from build123d import *
from OCP.BRepFilletAPI import BRepFilletAPI_MakeChamfer

# Parameters (mm, degrees)
SKETCH1_R           = 1.5
BOSS_EXTRUDE1_DEPTH = 3
BOSS_EXTRUDE2_START = 22.5
SKETCH2_W           = 3.5
SKETCH2_H           = 6
BOSS_EXTRUDE2_DEPTH = 29
SKETCH4_R           = 1.5
BOSS_EXTRUDE5_DEPTH = 1
CHAMFER2_SIZE       = 2
CHAMFER2_SIZE2      = 3.464101615
SKETCH3_W           = 24
SKETCH3_H           = 29
SKETCH3_R           = 11
BOSS_EXTRUDE4_DEPTH = 7
CHAMFER3_SIZE       = 2
MIRROR1_START       = 18
MIRROR1_OUTLINE_R   = 1.5
MIRROR1_DEPTH       = 4
MIRROR1_START_2     = -12
MIRROR1_2_DEPTH     = 6
MIRROR1_START_3     = 6
MIRROR1_3_DEPTH     = 6
MIRROR1_START_4     = 25.102290732
MIRROR1_4_OUTLINE_W = 2
MIRROR1_4_OUTLINE_H = 18.102290732
MIRROR1_4_DEPTH     = 1.897709268
MIRROR1_START_5     = 7.071067812
MIRROR1_5_OUTLINE_W = 2
MIRROR1_5_OUTLINE_H = 2.897709268
MIRROR1_5_DEPTH     = 3.889087296


with BuildPart() as part:
    # Sketch1 → Boss-Extrude1 (new body)
    with BuildSketch(Plane(origin=(0, 0, 0), x_dir=(1, 0, 0), z_dir=(0, 1, 0))):
        Polygon((-6, 17), (-3, 20), (3, 20), (6, 17), (6, -17), (3, -20), (-3, -20), (-6, -17), align=None)
        with Locations(Location((0, 14, 0), (0, 0, 270))):
            Circle(SKETCH1_R, mode=Mode.SUBTRACT)
        with Locations(Location((0, -14, 0), (0, 0, 270))):
            Circle(SKETCH1_R, mode=Mode.SUBTRACT)
    extrude(amount=BOSS_EXTRUDE1_DEPTH)

    # Sketch2 → Boss-Extrude2 (add)
    with BuildSketch(Plane(origin=(0, 3, 0), x_dir=(1, 0, 0), z_dir=(0, 1, 0)).offset(BOSS_EXTRUDE2_START)):
        with Locations((-7.75, 9)):
            Rectangle(SKETCH2_W, SKETCH2_H)
        with Locations((-7.75, -9)):
            Rectangle(SKETCH2_W, SKETCH2_H)
    extrude(amount=-BOSS_EXTRUDE2_DEPTH)

    # Sketch4 → Boss-Extrude5 (add)
    with BuildSketch(Plane(origin=(0, 3, 0), x_dir=(1, 0, 0), z_dir=(0, 1, 0))):
        Polygon((-3, 20), (-6, 17), (-6, 12), (-6, 6), (-6, -6), (-6, -12), (-6, -17), (-3, -20), (3, -20), (6, -17), (6, 17), (3, 20), align=None)
        with Locations(Location((0, 14, 0), (0, 0, 270))):
            Circle(SKETCH4_R, mode=Mode.SUBTRACT)
        with Locations(Location((0, -14, 0), (0, 0, 270))):
            Circle(SKETCH4_R, mode=Mode.SUBTRACT)
    extrude(amount=BOSS_EXTRUDE5_DEPTH)

    # Chamfer2: one chamfer whose edges measure the first distance from different faces: ONE call of the kernel's chamfer builder (chamfer() names one face for all edges)
    chamfer2_edges_1 = [part.edges().sort_by_distance(p)[0] for p in [
        (-6, 0, -9),
        (-6, 0, 9),
    ]]
    chamfer2_side_1 = [part.faces().sort_by_distance(p)[0] for p in [
        (0, 0, 0),
    ]]
    chamfer2_edges_2 = [part.edges().sort_by_distance(p)[0] for p in [
        (-6, 4, -9),
        (-6, 4, 9),
    ]]
    chamfer2_side_2 = [part.faces().sort_by_distance(p)[0] for p in [
        (0, 4, 0),
    ]]
    chamfer2 = BRepFilletAPI_MakeChamfer(part.part.solid().wrapped)
    for e in chamfer2_edges_1:
        chamfer2.Add(CHAMFER2_SIZE, CHAMFER2_SIZE2, e.wrapped, chamfer2_side_1[0].wrapped)  # the first distance lies on this face
    for e in chamfer2_edges_2:
        chamfer2.Add(CHAMFER2_SIZE, CHAMFER2_SIZE2, e.wrapped, chamfer2_side_2[0].wrapped)  # the first distance lies on this face
    add(Compound.cast(chamfer2.Shape()), mode=Mode.REPLACE)

    # Sketch3 → Boss-Extrude4 (add)
    with BuildSketch(Plane.ZY.offset(9.5)):
        with Locations((0, 11)):
            Rectangle(SKETCH3_W, SKETCH3_H)
        with Locations(Location((0, 11, 0), (0, 0, 236.944268849))):
            Circle(SKETCH3_R, mode=Mode.SUBTRACT)
    extrude(amount=BOSS_EXTRUDE4_DEPTH)

    # Chamfer3
    chamfer3_edges = [part.edges().sort_by_distance(p)[0] for p in [
        (-11.25, 25.5, -12),
        (-11.25, -3.5, -12),
        (-11.25, -3.5, 12),
        (-11.25, 25.5, 12),
    ]]
    chamfer(chamfer3_edges, length=CHAMFER3_SIZE)

    # Mirror1: read off the stored shape, not the designer's step
    # Mirror1 outline → Mirror1 (add)
    with BuildSketch(Plane(origin=(0, 0, 0), x_dir=(1, 0, 0), z_dir=(0, 1, 0)).offset(MIRROR1_START)):
        Polygon((-6, 17), (-6, 6), (-6, -6), (-6, -17), (-3, -20), (3, -20), (6, -17), (6, 17), (3, 20), (-3, 20), align=None)
        with Locations((0, -14)):
            Circle(MIRROR1_OUTLINE_R, mode=Mode.SUBTRACT)
        with Locations((0, 14)):
            Circle(MIRROR1_OUTLINE_R, mode=Mode.SUBTRACT)
    extrude(amount=MIRROR1_DEPTH)

    # Mirror1 2 outline → Mirror1 2 (add)
    with BuildSketch(Plane.XY.offset(MIRROR1_START_2)):
        Polygon((-6, 14.535898385), (-4, 18), (-6, 18), align=None)
        Polygon((-4, 22), (-6, 25.464101615), (-6, 22), align=None)
    extrude(amount=MIRROR1_2_DEPTH)

    # Mirror1 3 outline → Mirror1 3 (add)
    with BuildSketch(Plane.XY.offset(MIRROR1_START_3)):
        Polygon((-2.535898385, 18), (-6, 18), (-6, 16), align=None)
        Polygon((-4, 22), (-6, 25.464101615), (-6, 22), align=None)
    extrude(amount=MIRROR1_3_DEPTH)

    # Mirror1 4 outline → Mirror1 4 (cut)
    with BuildSketch(Plane(origin=(0, 0, 0), x_dir=(1, 0, 0), z_dir=(0, 0.7071067811865466, 0.7071067811865486)).offset(MIRROR1_START_4)):
        with Locations((-5, 16.051145366)):
            Rectangle(MIRROR1_4_OUTLINE_W, MIRROR1_4_OUTLINE_H)
    extrude(amount=MIRROR1_4_DEPTH, mode=Mode.SUBTRACT)

    # Mirror1 5 outline → Mirror1 5 (cut)
    with BuildSketch(Plane(origin=(0, 0, 0), x_dir=(1, 0, 0), z_dir=(0, 0.7071067811865466, 0.7071067811865486)).offset(MIRROR1_START_5)):
        with Locations((-5, 26.551145366)):
            Rectangle(MIRROR1_5_OUTLINE_W, MIRROR1_5_OUTLINE_H)
    extrude(amount=MIRROR1_5_DEPTH, mode=Mode.SUBTRACT)


solid = part.part
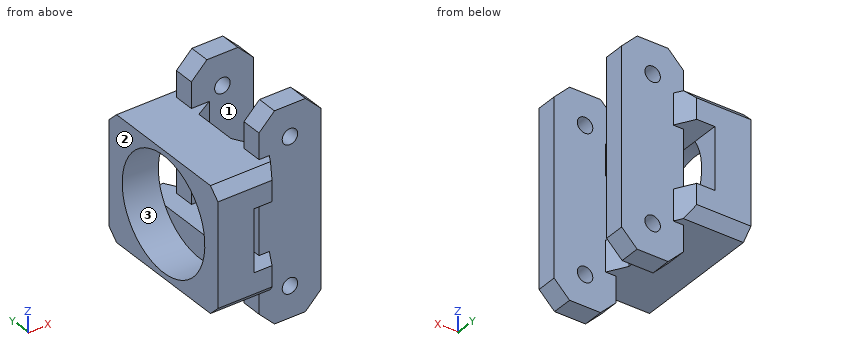
The model under review builds one solid part; all positions refer to its coordinate system, in mm. Face numbers are marked on the shaded views. A direction names the side the tool comes from. Round coordinates to 2 decimals unless told otherwise and drop trailing zeros. Order: outer loops, then holes, each group sorted by start corner. A loop starts at its lowest first (then second) coordinate and runs counter-clockwise, first axis right, second up. Notation, with made-up numbers: (87.25, -10) -> (125.25, -10) arc R11 ccw to (125.25, 11) -> close; hole circle Ø11 at (-33.75, 29.5). An arc over 180 degrees is marked (long way). Write item = value, one per line. Start each with the question number.
Item 1: Clearance check with flat-ended pins moving along their axes: pin 1 Ø8 at (x, y) = (-8, 1.5) entering from +Z; pin 2 Ø4 at (y, z) = (18, -15.5) entering from -X; pin 3 Ø4 at (x, z) = (0, 14) entering from +Y; pin 4 Ø4 at (y, z) = (7.5, 0) entering from -X. State where each tip first meets the part, or that it passes through.
Item 2: For line 1 along Z through (x, y) = (0, 19.7); line 2 along Y through (x, z) = (5, 10); line 3 along X through (y, z) = (1.7, -14), list the stretches that pass through material, from the lowest coordinate up.
Item 3: Consider section D-D on y = 13.5. Write out the cut boundary in (x, z).
Item 4: Consider section B-B on x = 2.5. Write out the cut boundary in (y, z).
Item 5: Consider section A-A on z = -16. Write out the cut boundary in (x, y).
Item 6: For the marked faces 1, 2 and 3, list the 3-axis set-ups (+Z, -Z, +X, -X, +Y, -Y) from which the entire face can be reached by the end or side of a thin tool; tool diameter is ignored.
Item 7: Consider section C-C on z = 0. Write out the cut boundary in (x, y), plus the area to 3 significant figures.
Conclusion:
q1.pin_1 = 19
q1.pin_2 = -6
q1.pin_3 = 22
q1.pin_4 = through
q2.line_1 = -20 to -15.5, -12.5 to 12.5, 15.5 to 20
q2.line_2 = 0 to 4, 18 to 22
q2.line_3 = -6 to -1.5, 1.5 to 6
q3.outline = (-16.5, -12) -> (-6, -12) -> (-6, -6) -> (-9.5, -6) -> (-9.5, -10.71) -> (-16.5, -10.71) -> close; (-16.5, 10.71) -> (-9.5, 10.71) -> (-9.5, 6) -> (-6, 6) -> (-6, 12) -> (-16.5, 12) -> close
q4.outline = (0, -20) -> (4, -20) -> (4, 20) -> (0, 20) -> close; (18, -20) -> (22, -20) -> (22, 20) -> (18, 20) -> close
q5.outline = (-6, 0) -> (6, 0) -> (6, 4) -> (-6, 4) -> close; (-6, 18) -> (6, 18) -> (6, 22) -> (-6, 22) -> close
q6.face_1 = +X
q6.face_2 = +Z, -Z, -X, +Y, -Y
q6.face_3 = -X
q7.outline = (-16.5, -3.5) -> (-9.5, -3.5) -> (-9.5, 0) -> (-16.5, 0) -> close; (-16.5, 22) -> (-9.5, 22) -> (-9.5, 25.5) -> (-16.5, 25.5) -> close; (-6, 0) -> (6, 0) -> (6, 4) -> (-6, 4) -> close; (-6, 18) -> (6, 18) -> (6, 22) -> (-6, 22) -> close
q7.area = 145 mm2
